from build123d import *

# Parameters (mm, degrees)
F0_W        = 40
F0_H        = 40
F1_DEPTH    = 20
F2_T        = -2
F3_T1_DEPTH = 207.7346390373
F4_R        = 5


# Not quite as in the source:
# - a fillet or chamfer that OpenCascade refuses, or shapes differently, is made with other operations: its cross-section is extruded or revolved along the edge and cut away or added


with BuildPart() as f1:
    # F0 (on Top) → F1 (new body)
    with BuildSketch(Plane.XY):
        Rectangle(F0_W, F0_H)
    extrude(amount=F1_DEPTH)

    # F2
    f2_openings = [f1.faces().sort_by_distance(p)[0] for p in [
        (20, 0, 10),
        (0, 20, 10),
    ]]
    offset(amount=F2_T, openings=f2_openings)

    # F3: chamfer of 40 on 6 edges, made by hand

    # F3_s2 → F3_t1 (cut)
    with BuildSketch(Plane.XY.offset(-102.8673195186)):
        Polygon((20, -20), (-20, 20), (20, 20), align=None)
    extrude(amount=F3_T1_DEPTH, mode=Mode.SUBTRACT)

    # F4
    f4_edges = [f1.edges().sort_by_distance(p)[0] for p in [
        (-20, -20, 10),
    ]]
    fillet(f4_edges, radius=F4_R)


solid = f1.part
Verification items for the finished model (mm, model axes). A direction names the side the tool comes from. Round coordinates to 2 decimals unless told otherwise and drop trailing zeros. Loops run counter-clockwise (first coordinate to the right, second up) from the corner with the lowest first, then second, coordinate; pieces in that order, holes last. Notation, with made-up numbers: (64, 79.5) - (103, 79.5) arc R31 ccw to (103, 117.5) - close; hole circle Ø9 at (40, 12.5). An arc over 180 degrees is marked (long way). Use one line per item in the form item = value.
1. Scan lines: probe 1 along Z at (x, y) = (-15.5, -15); probe 2 along X at (y, z) = (9, 7.5). Record each from-to range of solid material in increasing order.
A:
probe_1 = 0 to 2, 18 to 20
probe_2 = -20 to -18
2. Section check B-B on y = -2. Record the cut outline in (x, z), and give its area (3 significant figures).
A:
outline = (-20, 0) - (2, 0) - (2, 2) - (-18, 2) - (-18, 18) - (2, 18) - (2, 20) - (-20, 20) - close
area = 120 mm²
3. Section check C-C on z = 9.25. Record the cut outline in (x, y), and give its area (3 significant figures).
A:
outline = (-20, -15) arc R5 ccw to (-15, -20) - (20, -20) - (18, -18) - (-18, -18) - (-18, 18) - (-20, 20) - close
area = 147 mm²
4. Access from +Z, -Z, +X, -X, +Y, -Y to the whole of each face (thin tool, end or side, straight path). Record for faces 5 (the flat face through (-18, 0, 10)), 6 (the flat face through (2, -20, 10)).
A:
face_5 = +X, +Y
face_6 = +Z, -Z, +X, -X, -Y
5. Section check A-A on x = -6.5. Record the cut outline in (y, z).
A:
outline = (-20, 0) - (6.5, 0) - (6.5, 2) - (-18, 2) - (-18, 18) - (6.5, 18) - (6.5, 20) - (-20, 20) - close
6. Draft check along Z on faces 1 (the flat face through (-9, -9, 0)), 2 (the flat face through (0.1, -0.1, 1.8)), 3 (the flat face through (0, -18, 10)), 4 (the flat face through (-8, -8, 2)). Enter one of: pulls with the +Z half, pulls with the -Z half, needs draft (parallel to the pull), parting line crosses it, or undercut.
A:
face_1 = pulls with the -Z half
face_2 = needs draft
face_3 = undercut
face_4 = undercut
7. Gauge pin test, flat ends, axial feed: pin 1 Ø8 at (x, z) = (-2.5, 13) entering from +Y; pin 2 Ø11 at (x, y) = (4.5, 7) entering from +Z; pin 3 Ø8 at (y, z) = (-7, 9) entering from +X. Record the tip position at first contact, or that the pin passes through.
A:
pin_1 = -18
pin_2 = through
pin_3 = -18
